The model under review builds one solid part; all positions refer to its coordinate system, in mm. Face numbers are marked on the shaded views. A direction names the side the tool comes from. Give positions to 0.01 mm unless a question says otherwise; leave off trailing zeros. Order: outer loops, then holes, each group sorted by start corner. A loop starts at its lowest first (then second) coordinate and runs counter-clockwise, first axis right, second up.
Solid Edge part; units mm, degrees
sketch "Sketch1" plane through (0, 0, 0) normal (0, 0, 1) x (1, 0, 0)
  circle A0 centre (0, 0) radius 8
extrude "Protrusion1" add sketch "Sketch1" along normal blind 10.5
sketch "Sketch2" plane through (0, 0, 10.5) normal (0, 0, 1) x (0, 1, 0)
  circle A0 centre (0, 0) radius 9.35
extrude "Extrusionsausprägung_2" add sketch "Sketch2" along normal blind 2
sketch "Sketch3" plane through (0, 0, 12.5) normal (0, 0, 1) x (0, 1, 0)
  circle A0 centre (0, 0) radius 10.5
extrude "Extrusionsausprägung_3" add sketch "Sketch3" along normal blind 11
sketch "Sketch4" plane through (0, 0, 17.5) normal (0, 0, 1) x (0, 1, 0)
  circle A0 centre (0, 0) radius 10.9
extrude "Extrusionsausprägung_4" add sketch "Sketch4" along normal blind 3
sketch "Sketch5" plane through (0, -10.5, 0) normal (0, -1, 0) x (1, 0, 0)
  line L0 (0, 23.5) -> (2.5, 23.5)
  line L1 (2.5, 23.5) -> (2.5, 12.5)
  line L2 (2.5, 12.5) -> (-2.5, 12.5)
  line L3 (-2.5, 12.5) -> (-2.5, 23.5)
  line L4 (-2.5, 23.5) -> (0, 23.5)
extrude "Extrusionsausprägung_5" add sketch "Sketch5" along normal mid plane 0.8
sketch "Sketch6" plane through (0, 10.5, 0) normal (0, -1, 0) x (1, 0, 0)
  line L0 (-2.5, 23.5) -> (2.5, 23.5)
  line L1 (2.5, 23.5) -> (2.5, 12.5)
  line L2 (2.5, 12.5) -> (-2.5, 12.5)
  line L3 (-2.5, 12.5) -> (-2.5, 23.5)
extrude "Extrusionsausprägung_6" add sketch "Sketch6" along normal mid plane 0.8
sketch "Sketch7" plane through (0, 0, 23.5) normal (0, 0, 1) x (0, 1, 0)
  circle A0 centre (0, 0) radius 10.4
extrude "Extrusionsausprägung_7" add sketch "Sketch7" along normal mid plane 2
sketch "Sketch8" plane through (0, 0, 0) normal (1, 0, 0) x (0, 1, 0)
  line L0 (0, 23.5) -> (10.4, 23.5)
  line L1 (10.4, 23.5) -> (10.4, 35.5)
  arc A0 (10.4, 35.5) -> (9.4, 36.5) centre (9.4, 35.5) ccw
  line L2 (9.4, 36.5) -> (-13.6, 36.5)
  arc A1 (-14.6, 35.5) -> (-13.6, 36.5) centre (-13.6, 35.5) cw
  line L3 (-14.6, 35.5) -> (-14.6, 26)
  arc A2 (-14.6, 26) -> (-13.6, 25) centre (-13.6, 26) ccw
  line L4 (-13.6, 25) -> (-10.9, 25)
  arc A3 (-10.9, 25) -> (-10.4, 24.5) centre (-10.9, 24.5) cw
  line L5 (-10.4, 23.5) -> (-10.4, 24.5)
  line L6 (0, 23.5) -> (-10.4, 23.5)
extrude "Extrusionsausprägung_10" add sketch "Sketch8" along normal mid plane 1.5
sketch "Sketch9" plane through (0, 0, 0) normal (0, -1, 0) x (1, 0, 0)
  line L0 (22.5, 7) -> (22.5, 8)
  line L1 (22.5, 8) -> (22.0581, 8.5)
  line L2 (19.5, 9) -> (22.0581, 8.5)
  line L3 (19.5, 8) -> (19.5, 9)
  line L4 (14.5, 9) -> (19.5, 8)
  line L5 (14.5, 9) -> (14.5, 8)
  line L6 (14.5, 8) -> (5.2197, 10.1408)
  line L7 (5.2197, 10.1408) -> (-5.572, 10.0596)
  line L8 (-14.5, 8) -> (-5.572, 10.0596)
  line L9 (-14.5, 8) -> (-14.5, 9)
  line L10 (-14.5, 9) -> (-19.5, 8)
  line L11 (-19.5, 8) -> (-19.5, 9)
  line L12 (-19.5, 9) -> (-22.1628, 8.5)
  line L13 (-22.1628, 8.5) -> (-22.5, 8)
  line L14 (-22.5, 7) -> (-22.5, 8)
  line L15 (-22.5, 7) -> (22.5, 7)
revolve "RevolvedProtrusion1" add sketch "Sketch9" angle 360 about axis through (0, 0, 5) along (1, 0, 0)
sketch "Sketch10" plane through (22.5, 0, 5) normal (1, 0, 0) x (0, 1, 0)
  circle A0 centre (0, 0) radius 2
extrude "Cutout1" cut sketch "Sketch10" against normal blind 49.253
sketch "Sketch11" plane through (0, 0, 0) normal (0, 0, -1) x (1, 0, 0)
  line L0 (-1.7342, 3.7694) -> (-7.0229, 0.602)
  line L1 (-7.0229, 0.602) -> (-5.7187, -2.8522)
  line L2 (-5.7187, -2.8522) -> (2.9095, -3.9271)
  line L3 (2.9095, -3.9271) -> (6.9799, -0.516)
  line L4 (6.9799, -0.516) -> (4.9447, 3.4971)
  line L5 (4.9447, 3.4971) -> (-1.7342, 3.7694)
extrude "Extrusionsausschnitt_2" cut sketch "Sketch11" along normal blind 1.4314
sketch "Sketch12" plane through (0, 0, 0) normal (0, 0, -1) x (1, 0, 0)
  circle A0 centre (-2.8, 0) radius 4.7
extrude "Protrusion2" add sketch "Sketch12" along normal mid plane 3.5
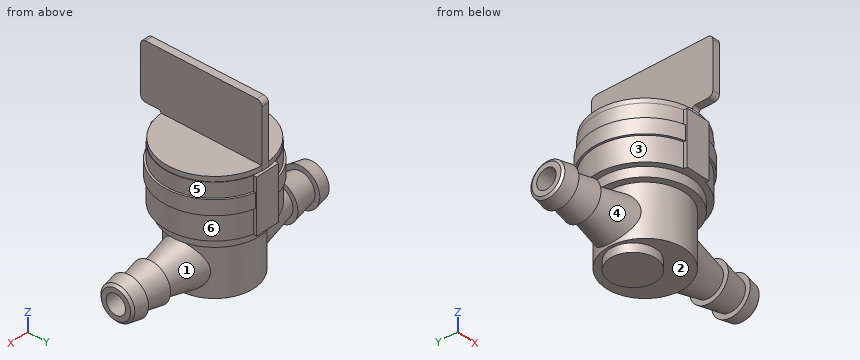
Item 1: Take a section at C-C (x = -13). Give the boundary of the cut face in (y, z).
Values found:
outline: circle Ø6.69 at (0, 5); hole circle Ø4 at (0, 5)
Item 2: Take a section at B-B (x = 0). Give the boundary of the cut face in (y, z).
Values found:
outline: (-14.6, 26) arc R1 ccw to (-13.6, 25) - (-10.9, 25) arc R0.5 cw to (-10.4, 24.5) - (-10.4, 23.5) - (-10.9, 23.5) - (-10.9, 12.5) - (-9.35, 12.5) - (-9.35, 10.5) - (-8, 10.5) - (-8, 0) - (-3.77, 0) - (-3.77, -1.75) - (3.77, -1.75) - (3.77, 0) - (8, 0) - (8, 10.5) - (9.35, 10.5) - (9.35, 12.5) - (10.9, 12.5) - (10.9, 23.5) - (10.4, 23.5) - (10.4, 35.5) arc R1 ccw to (9.4, 36.5) - (-13.6, 36.5) arc R1 ccw to (-14.6, 35.5) - close; hole circle Ø4 at (0, 5)
Item 3: Draft analysis for pull direction X (two halves, no side actions). For the marked faces 1, 2 and 3, state which applies: released by +X, released by -X, zero draft, split by the parting line, or undercut.
Values found:
face 1: undercut
face 2: zero draft
face 3: released by -X
Item 4: For line 1 (Z direction, x = -4, y = 0); line 2 (Z direction, x = -9.5, y = 1); line 3 (Z direction, x = 8.5, y = 0), list the stretches that pass through material, from the lowest coordinate up.
Values found:
line 1: z = -1.75 to 3, 7 to 24.5
line 2: z = 0.97 to 3.27, 6.73 to 9.03, 12.5 to 24.5
line 3: z = 0.62 to 3, 7 to 9.38, 10.5 to 24.5
Item 5: For the marked faces 4, 5 and 6, list the 3-axis set-ups (+Z, -Z, +X, -X, +Y, -Y) from which the entire face can be reached by the end or side of a thin tool; tool diameter is ignored.
Values found:
face 4: none
face 5: +Z, +X
face 6: +X
Item 6: Take a section at A-A (z = 16). Give the boundary of the cut face in (x, y).
Values found:
outline: (-2.5, -10.9) - (2.5, -10.9) - (2.5, -10.2) arc R10.5 ccw to (2.5, 10.2) - (2.5, 10.9) - (-2.5, 10.9) - (-2.5, 10.2) arc R10.5 ccw to (-2.5, -10.2) - close
Item 7: Clearance check with flat-ended pins moving along their axes: pin 1 Ø2.5 at (x, y) = (-8.5, -4) entering from -Z; pin 2 Ø9 at (x, y) = (8, 3) entering from +Z; pin 3 Ø4 at (y, z) = (-6.5, 25.5) entering from +X. State where each tip first meets the part, or that it passes through.
Values found:
pin 1: stops at z = 1.52
pin 2: stops at z = 24.5
pin 3: stops at x = 9.24
